```python
from build123d import *

# Parameters (mm, degrees)
SKETCH1_R                            = 20
BOSS_EXTRUDE1_DEPTH                  = 10
SKETCH1_R_2                          = 40
SKETCH1_R_3                          = 35
BOSS_EXTRUDE1_2_DEPTH                = 10
BOSS_EXTRUDE2_REACH                  = 89.446
BOSS_EXTRUDE2_END_RADIUS             = 35
BOSS_EXTRUDE2_START                  = 30
BOSS_EXTRUDE2_DIRECTION_2_REACH      = 89.446
BOSS_EXTRUDE2_DIRECTION_2_END_RADIUS = 20
CIRPATTERN1_COUNT                    = 12
SKETCH5_R                            = 3.167731354
BOSS_EXTRUDE3_DEPTH                  = 10
SCALE1_SCALE                         = 0.75


with BuildPart() as part:
    # Sketch1 → Boss-Extrude1 (new body)
    with BuildSketch(Plane(origin=(0, 0, 0), x_dir=(1, 0, 0), z_dir=(0, 1, 0))):
        with Locations(Location((0, 0, 0), (0, 0, 270))):
            Circle(SKETCH1_R)
    extrude(amount=BOSS_EXTRUDE1_DEPTH)


with BuildPart() as body_2:
    # Sketch1 → Boss-Extrude1 2 (new body)
    with BuildSketch(Plane(origin=(0, 0, 0), x_dir=(1, 0, 0), z_dir=(0, 1, 0))):
        with Locations(Location((0, 0, 0), (0, 0, 270))):
            Circle(SKETCH1_R_2)
        with Locations(Location((0, 0, 0), (0, 0, 270))):
            Circle(SKETCH1_R_3, mode=Mode.SUBTRACT)
    extrude(amount=BOSS_EXTRUDE1_2_DEPTH)


    add(part.part)  # Boss-Extrude2 merges part
    # Boss-Extrude2: up to this cylinder (the profile starts inside it)
    boss_extrude2_end = Plane(origin=(0, 5, 0), z_dir=(0, -1, 0)) * Cylinder(BOSS_EXTRUDE2_END_RADIUS, 249.892, mode=Mode.PRIVATE)
    # Sketch4 → Boss-Extrude2 (add, up to the surface)
    with BuildSketch(Plane(origin=(0, 0, 0), x_dir=(0, 0, -1), z_dir=(1, 0, 0)).offset(BOSS_EXTRUDE2_START), mode=Mode.PRIVATE) as boss_extrude2_sk1:
        Polygon((-4.262410526, 0), (4.031443844, 10), (5.315133993, 10), (-2.978720377, 0), align=None)
    boss_extrude2_tool1 = extrude(boss_extrude2_sk1.sketch, amount=BOSS_EXTRUDE2_REACH, mode=Mode.PRIVATE) & boss_extrude2_end
    boss_extrude2 = boss_extrude2_tool1.solids().sort_by_distance((30, 5, -0.526362))[0]
    add(boss_extrude2)

    # Boss-Extrude2 direction 2: up to this cylinder (the profile starts outside it)
    boss_extrude2_direction_2_end = Plane(origin=(0, 5, 0), z_dir=(0, -1, 0)) * Cylinder(BOSS_EXTRUDE2_DIRECTION_2_END_RADIUS, 219.892, mode=Mode.PRIVATE)
    # Sketch4 → Boss-Extrude2 direction 2 (add, up to the surface)
    with BuildSketch(Plane(origin=(0, 0, 0), x_dir=(0, 0, -1), z_dir=(1, 0, 0)).offset(BOSS_EXTRUDE2_START), mode=Mode.PRIVATE) as boss_extrude2_direction_2_sk1:
        Polygon((-4.262410526, 0), (4.031443844, 10), (5.315133993, 10), (-2.978720377, 0), align=None)
    boss_extrude2_direction_2_tool1 = extrude(boss_extrude2_direction_2_sk1.sketch, amount=-BOSS_EXTRUDE2_DIRECTION_2_REACH, mode=Mode.PRIVATE) - boss_extrude2_direction_2_end
    boss_extrude2_direction_2 = boss_extrude2_direction_2_tool1.solids().sort_by_distance((30, 5, -0.526362))[0]
    add(boss_extrude2_direction_2)
    boss_extrude2 = boss_extrude2 + boss_extrude2_direction_2  # both directions under the feature's name, for the pattern or mirror that repeats it

    # CirPattern1: Boss-Extrude2 ×12 about axis
    cirpattern1_axis = Axis((0, 0, 0), (0, 1, 0))
    for i in range(1, CIRPATTERN1_COUNT):
        add(boss_extrude2.rotate(cirpattern1_axis, i * 360 / CIRPATTERN1_COUNT))

    # Sketch5 → Boss-Extrude3 (add)
    with BuildSketch(Plane(origin=(0, 10, 0), x_dir=(1, 0, 0), z_dir=(0, 1, 0))):
        with Locations(Location((0, 0, 0), (0, 0, 270))):
            Circle(SKETCH5_R)
    extrude(amount=BOSS_EXTRUDE3_DEPTH)


with BuildPart() as body_2_1:
    # Scale1: scaled about (0, 0, 0)
    add(body_2.part.scale(SCALE1_SCALE))


solid = body_2_1.part
```
Work out the finished part from the listing and answer in its coordinate system (mm). A direction names the side the tool comes from. Give positions to 0.01 mm unless a question says otherwise; leave off trailing zeros. Order: outer loops, then holes, each group sorted by start corner. A loop starts at its lowest first (then second) coordinate and runs counter-clockwise, first axis right, second up.
1. Section D-D, the plane x = -12.5 is taken. Determine the outline of the cut face in (y, z).
Result sheet:
outline: (0, -27.27) - (7.5, -27.27) - (7.5, -23.08) - (2.99, -23.08) - (7.5, -15.6) - (7.5, -13.68) - (1.83, -23.08) - (0, -23.08) - close; (0, -10.91) - (2.73, -8.29) - (7.5, -8.29) - (7.5, 8.29) - (4.98, 8.29) - (7.5, 10.71) - (7.5, 11.82) - (3.82, 8.29) - (0, 8.29) - (0, -8.29) - (1.57, -8.29) - (0, -9.8) - close; (0, 15.26) - (4.72, 23.08) - (7.5, 23.08) - (7.5, 27.27) - (0, 27.27) - (0, 23.08) - (3.56, 23.08) - (0, 17.18) - close
2. Straight lines are drawn through the part: L1, parallel to X at y = 3.5, z = 19.5; L2, parallel to Z at x = 22, y = 0.75; L3, parallel to X at y = 2.75, z = 4. For each, find the intervals that lie inside material, in ascending order.
Result sheet:
L1: x = -22.8 to -17.57, -11.6 to -10.49, -0.29 to 0.67, 10.92 to 12.03, 17.57 to 22.8
L2: z = -20.4 to -14.32, -10.84 to -9.73, 1.61 to 2.57, 14.32 to 20.4
L3: x = -29.73 to -25.94, -14.46 to 14.46, 25.94 to 29.73
3. Section B-B, the plane x = -18.5 is taken. Determine the outline of the cut face in (y, z).
Result sheet:
outline: (0, -23.62) - (7.5, -23.62) - (7.5, -18.62) - (0, -18.62) - close; (0, -14.37) - (7.5, -7.19) - (7.5, -6.08) - (0, -13.26) - close; (0, -3.2) - (7.5, 3.02) - (7.5, 3.99) - (0, -2.23) - close; (0, 6.99) - (7.5, 14.17) - (7.5, 15.28) - (0, 8.1) - close; (0, 18.62) - (7.5, 18.62) - (7.5, 23.62) - (0, 23.62) - close
4. The mould has two halves that part along X. Classify faces 1 (the cylindrical face through (0.714, 11.198, 2.266)), 2 (the cylindrical face through (-4.2, 3.7, -14.4)), 3 (the flat face through (0, 0, 0)): released by +X, released by -X, zero draft, split by the parting line, or undercut.
Result sheet:
face 1: split by the parting line
face 2: undercut
face 3: zero draft
5. Section A-A, the plane z = 19.5 is taken. Determine the outline of the cut face in (x, y).
Result sheet:
outline: (-22.8, 0) - (-17.57, 0) - (-17.57, 7.5) - (-22.8, 7.5) - close; (-14.95, 0) - (-13.84, 0) - (-6.66, 7.5) - (-7.77, 7.5) - close; (-3.2, 0) - (-2.23, 0) - (3.99, 7.5) - (3.02, 7.5) - close; (7.57, 0) - (8.68, 0) - (15.86, 7.5) - (14.75, 7.5) - close; (17.57, 0) - (22.8, 0) - (22.8, 7.5) - (17.57, 7.5) - close
6. For faces 4 (the flat face through (20.44, 3.8, -0.92)), 5 (the flat face through (-20.37, 3.7, -0.13)), 6 (the cylindrical face through (6.539, 3.698, -25.423)), determine the directions among +Z, -Z, +X, -X, +Y, -Y from which every point of the face is accessible in a straight line to the end or side of a thin tool.
Result sheet:
face 4: -Y
face 5: +Y
face 6: none
7. Section C-C, the plane z = 12.5 is taken. Determine the outline of the cut face in (x, y), and give its area (3 significant figures).
Result sheet:
outline: (-27.27, 0) - (-23.08, 0) - (-23.08, 1.83) - (-13.68, 7.5) - (-15.6, 7.5) - (-23.08, 2.99) - (-23.08, 7.5) - (-27.27, 7.5) - close; (-10.91, 0) - (-9.8, 0) - (-8.29, 1.57) - (-8.29, 0) - (8.29, 0) - (8.29, 3.82) - (11.82, 7.5) - (10.71, 7.5) - (8.29, 4.98) - (8.29, 7.5) - (-8.29, 7.5) - (-8.29, 2.73) - close; (15.26, 0) - (17.18, 0) - (23.08, 3.56) - (23.08, 0) - (27.27, 0) - (27.27, 7.5) - (23.08, 7.5) - (23.08, 4.72) - close
area: 211 mm2
8. Each of these flat-tipped pins is pushed along its axis until it touches: P1, Ø6, axis at x = 23, y = 6, coming from the -Z side; P2, Ø2, axis at y = 9, z = 10, coming from the +X side; P3, Ø2, axis at x = 11.5, z = -10.5, coming from the +Y side; P4, Ø4, axis at x = 3.5, z = -20.5, coming from the +Y side. Where does it stop, or does it pass through?
Result sheet:
P1: stops at z = -22.36
P2: passes through
P3: stops at y = 7.5
P4: stops at y = 2.05
